The model under review builds one solid part; all positions refer to its coordinate system, in mm. A direction names the side the tool comes from. Coordinates: 2 decimals unless noted, no trailing zeros. Loops run counter-clockwise (first coordinate to the right, second up) from the corner with the lowest first, then second, coordinate; pieces in that order, holes last. Notation, with made-up numbers: (71.25, 32) - (103.25, 32) arc R19 ccw to (103.25, 69) - close; hole circle Ø10 at (37, 85.25). An arc over 180 degrees is marked (long way). One line per item, written item: value. Start each with the question number.
1. For faces 4 (the face through (-33, -12, 5)), 5 (the face through (40, -12, 14)), 6 (the face through (33, -12, 5)), list the 3-axis set-ups (+Z, -Z, +X, -X, +Y, -Y) from which the entire face can be reached by the end or side of a thin tool; tool diameter is ignored.
2. We need section C-C, the plane x = -24. Give the boundary of the cut face in (y, z), then the cut area to 3 significant figures.
3. Mouldability with a two-part tool opening along Z and no side actions: class faces 1 (the face through (37.15, -12.32, 26.99)), 2 (the face through (38, -12, 6)), 3 (the face through (-1, -25, 0)) as +Z half, -Z half, draft (parallel to the pull), parting line (faces both ways), or undercut.
4. We need section A-A, the plane x = 20. Give the boundary of the cut face in (y, z).
5. We need section B-B, the plane y = -13.5. Give the boundary of the cut face in (x, z), then the cut area to 3 significant figures.
6. To check wall thickness, follow line 1 (Z direction, x = 20, y = -11.25); line 2 (X direction, y = -13.25, z = 0); line 3 (X direction, y = -13.75, z = -6.5). State the ranges of each line that lie inside material, in increasing order.
7. We need section D-D, the plane z = 0. Give the boundary of the cut face in (x, y).
8. Insertion check: P1, Ø6.5, axis at x = 34, y = -8, coming from the -Z side; P2, Ø3, axis at y = -20.5, z = -23, coming from the +X side. Each pin has a flat end and moves straight along its axis. Give the tip position at first contact, or say it passes through.
from build123d import *

# Parameters (mm, degrees)
F1_DEPTH = 25


with BuildPart() as f1:
    # F0 (on Front) → F1 (new body)
    with BuildSketch(Plane.XZ):
        with BuildLine():
            ThreePointArc((-28.660254, 5), (-10, 0), (-28.660254, -5))
            Line((-28.660254, -5), (-37, -5))
            Line((-37, -5), (-40, -8))
            Line((-40, -8), (-40, -20))
            ThreePointArc((-40, -20), (-37.071068, -27.071068), (-30, -30))
            Line((-30, -30), (0, -30))
            Line((0, -30), (30, -30))
            ThreePointArc((30, -30), (37.071068, -27.071068), (40, -20))
            Line((40, -20), (40, -8))
            Line((40, -8), (37, -5))
            Line((37, -5), (28.660254, -5))
            ThreePointArc((28.660254, -5), (10, 0), (28.660254, 5))
            Line((28.660254, 5), (37, 5))
            Line((37, 5), (40, 8))
            Line((40, 8), (40, 20))
            ThreePointArc((40, 20), (37.071068, 27.071068), (30, 30))
            Line((30, 30), (0, 30))
            Line((0, 30), (-30, 30))
            ThreePointArc((-30, 30), (-37.071068, 27.071068), (-40, 20))
            Line((-40, 20), (-40, 8))
            Line((-40, 8), (-37, 5))
            Line((-37, 5), (-28.660254, 5))
        make_face()
    extrude(amount=F1_DEPTH)


solid = f1.part
Findings below:
1. face 4: -X, +Y, -Y
1. face 5: +Z, -Z, +X, +Y, -Y
1. face 6: +X, +Y, -Y
2. outline: (-25, -30) - (0, -30) - (0, -9.17) - (-25, -9.17) - close; (-25, 9.17) - (0, 9.17) - (0, 30) - (-25, 30) - close
2. area: 1,040 mm2
3. face 1: +Z half
3. face 2: undercut
3. face 3: draft
4. outline: (-25, -30) - (0, -30) - (0, -10) - (-25, -10) - close; (-25, 10) - (0, 10) - (0, 30) - (-25, 30) - close
5. outline: (-40, -20) arc R10 ccw to (-30, -30) - (30, -30) arc R10 ccw to (40, -20) - (40, -8) - (37, -5) - (28.66, -5) arc R10 cw (long way) to (28.66, 5) - (37, 5) - (40, 8) - (40, 20) arc R10 ccw to (30, 30) - (-30, 30) arc R10 ccw to (-40, 20) - (-40, 8) - (-37, 5) - (-28.66, 5) arc R10 cw (long way) to (-28.66, -5) - (-37, -5) - (-40, -8) - close
5. area: 3,860 mm2
6. line 1: -30 to -10, 10 to 30
6. line 2: -10 to 10
6. line 3: -38.5 to -27.6, -12.4 to 12.4, 27.6 to 38.5
7. outline: (-10, -25) - (10, -25) - (10, 0) - (-10, 0) - close
8. P1: z = -29.97
8. P2: x = 39.89
